from build123d import *


with BuildPart() as part:
    # Croquis1 one side → Revolución1 (revolve)
    with BuildSketch(Plane(origin=(0, 0, 0), x_dir=(0, 0, -1), z_dir=(1, 0, 0))):
        Polygon((-45, 106), (-45, 150), (-50.5, 150), (-50.5, 25.75), (50.5, 25.75), (50.5, 150), (45, 150), (45, 106), align=None)
    revolve(axis=Axis((0, 0, 50.5), (0, 0, -1)))


solid = part.part
Design review of the part built by this model. Coordinates are the model's own, in mm. A direction names the side the tool comes from. Round coordinates to 2 decimals unless told otherwise and drop trailing zeros. Order: outer loops, then holes, each group sorted by start corner. A loop starts at its lowest first (then second) coordinate and runs counter-clockwise, first axis right, second up. Notation, with made-up numbers: M -40,57.25 L -2,57.25 A28 ccw -2,85.25 Z; hole C -21.75,-17.75 d4. An arc over 180 degrees is marked long. Answer as CSV lines item,"result". Start each with the question number.
1) Add section C-C (z = -30.5). Give the boundary of the cut face in (x, y), then the cut area to 3 significant figures.
2) Tool access review of faces 1 (the face through (148.724, -19.527, -47.712)), 2 (the face through (-31, -102, -45)): name each direction out of +Z, -Z, +X, -X, +Y, -Y from which nothing blocks a thin tool from reaching the whole face with its end or side.
3) For pin 1 Ø4 at (y, z) = (51.5, -38.5) entering from +X; pin 2 Ø2 at (x, z) = (-16, 9.5) entering from +Y; pin 3 Ø12 at (y, z) = (13.5, 32.5) entering from +X, all flat-tipped, find the tip position at first contact; note any pin that passes through.
4) The part is to be moulded in two halves that separate along Z. For faces 3 (the face through (-31, 102, 45)), 4 (the face through (148.724, -19.527, 47.788)), 5 (the face through (-31, 2, -50.5)), say which applies: +Z half, -Z half, draft (parallel to the pull), parting line (faces both ways), or undercut.
5) Add section A-A (x = 0). Give the boundary of the cut face in (y, z).
6) Wall thickness on line 1 along X through (y, z) = (0, -8); line 2 along Z through (x, y) = (-62, 99): over which ranges is each line inside the solid? List them lowest first. Write a range as [from, to].
7) Add section D-D (x = -111). Give the boundary of the cut face in (y, z), then the cut area to 3 significant figures.
Resolved:
1,outline,"C 0,0 d212; hole C 0,0 d51.5"
1,area,"33,200 mm^2"
2,face 1,"+Z, -Z"
2,face 2,"none"
3,pin 1,"x = 93.73"
3,pin 2,"y = 104.93"
3,pin 3,"x = 105.73"
4,face 3,"undercut"
4,face 4,"draft"
4,face 5,"-Z half"
5,outline,"M -150,-50.5 L -25.75,-50.5 L -25.75,50.5 L -150,50.5 L -150,45 L -106,45 L -106,-45 L -150,-45 Z; M 25.75,-50.5 L 150,-50.5 L 150,-45 L 106,-45 L 106,45 L 150,45 L 150,50.5 L 25.75,50.5 Z"
6,line 1,"[-106, -25.75], [25.75, 106]"
6,line 2,"[-50.5, -45], [45, 50.5]"
7,outline,"M -100.89,-50.5 L 100.89,-50.5 L 100.89,-45 L -100.89,-45 Z; M -100.89,45 L 100.89,45 L 100.89,50.5 L -100.89,50.5 Z"
7,area,"2,220 mm^2"
